The listing builds one solid part. Answer for the finished solid, in the listing's coordinates (mm). A direction names the side the tool comes from. Give positions to 0.01 mm unless a question says otherwise; leave off trailing zeros. Order: outer loops, then holes, each group sorted by start corner. A loop starts at its lowest first (then second) coordinate and runs counter-clockwise, first axis right, second up. Notation, with made-up numbers: (83, 53.5) - (115, 53.5) arc R6 cw to (115, 57.5) - close; hole circle Ø5 at (17, -8). An arc over 180 degrees is marked (long way). Write each question's results on one line, items separated by ' | '. Start each with the question number.
1. Section C-C (y = -38) is taken. Give the vertices of the cut face in (x, z).
2. Flat-ended cylindrical pins translate along their axes: pin 1 (4 mm diameter, centred on y = -10, z = 2.5, fed in from -X); pin 2 (5 mm diameter, centred on x = 0, y = -72.05, fed in from +Z); pin 3 (5 mm diameter, centred on x = 13, y = -22, fed in from +Z); pin 4 (6 mm diameter, centred on y = -20, z = -1, fed in from +X). Find the tip coordinate at first contact, or state that the pin passes through.
3. Section A-A (y = -15) is taken. Give the vertices of the cut face in (x, z).
4. Section B-B (x = -3) is taken. Give the vertices of the cut face in (y, z).
5. Find the intervals of material crossed by L1, parallel to Y at x = 0, z = 0.75; L2, parallel to Y at x = -15.5, z = 5; L3, parallel to Y at x = -8.5, z = -0.25, in increasing order.
6. Determine the mould class of faces 1 (the face through (-0.52, -68.08, -0.04)), 2 (the face through (2.305, -41.097, 0.035)), 3 (the face through (-19.33, -0.65, 0.04)), 4 (the face through (4, -33, -2.5)) for opening direction X: released by +X, released by -X, zero draft, split by the parting line, or undercut.
7. Which of the six approach directions +Z, -Z, +X, -X, +Y, -Y give full straight-line access (tool end or side, diameter ignored) to faces 5 (the face through (0.979, -37.367, 0.035)), 6 (the face through (-14, -9, 10)), 7 (the face through (-17.48, -8.8, 7.16))?
8. Section D-D (z = 3.5) is taken. State how many separate pieces and enclosed holes the cut face has, and give its area (3 significant figures).
from build123d import *

# Parameters (mm, degrees)
CROQUIS1_R              = 4
CROQUIS1_R_2            = 1.75
SALIENTE_EXTRUIR1_DEPTH = 2.5
CROQUIS1_3_R            = 2.5
CROQUIS1_3_R_2          = 1.75
SALIENTE_EXTRUIR2_DEPTH = 10
REDONDEO1_R             = 2
REDONDEO2_R             = 2


with BuildPart() as part:
    # Croquis1 → Saliente-Extruir1 (new, symmetric)
    with BuildSketch(Plane.XY):
        with BuildLine():
            Line((20.001432119, 0), (-20.001432119, 0))
            Line((-20.001432119, 0), (-14.963460754, -72.046347106))
            ThreePointArc((-14.963460754, -72.046347106), (0, -86), (14.963460754, -72.046347106))
            Line((14.963460754, -72.046347106), (20.001432119, 0))
        make_face()
        with Locations((0, -72.046347106)):
            Circle(CROQUIS1_R, mode=Mode.SUBTRACT)
        Polygon((12.515549555, -64.046347106), (-10.788577252, -64.046347106), (15.770666891, -17.496000466), align=None, mode=Mode.SUBTRACT)
        Polygon((-12.704099543, -61.349956664), (-16.011890152, -14.046347106), (14.28491785, -14.046347106), align=None, mode=Mode.SUBTRACT)
        with Locations((-15.5, -7.276347106)):
            Circle(CROQUIS1_R_2, mode=Mode.SUBTRACT)
        with Locations((15.5, -7.276347106)):
            Circle(CROQUIS1_R_2, mode=Mode.SUBTRACT)
    extrude(amount=SALIENTE_EXTRUIR1_DEPTH, both=True)

    # Croquis1_3 → Saliente-Extruir2 (add)
    # profile 1 of 2: a face of its own
    with BuildSketch(Plane.XY):
        with Locations((-15.5, -7.276347106)):
            Circle(CROQUIS1_3_R)
        with Locations((-15.5, -7.276347106)):
            Circle(CROQUIS1_3_R_2, mode=Mode.SUBTRACT)
    # profile 2 of 2: a face of its own
    with BuildSketch(Plane.XY):
        with Locations(Location((15.5, -7.276347106, 0), (0, 0, 180))):
            Circle(CROQUIS1_3_R)
        with Locations(Location((15.5, -7.276347106, 0), (0, 0, 180))):
            Circle(CROQUIS1_3_R_2, mode=Mode.SUBTRACT)
    extrude(amount=SALIENTE_EXTRUIR2_DEPTH)

    # Redondeo1
    redondeo1_edges = [part.edges().sort_by_distance(p)[0] for p in [
        (18, -7.276347106, 2.5),
        (-18, -7.276347106, 2.5),
    ]]
    fillet(redondeo1_edges, radius=REDONDEO1_R)

    # Redondeo2
    redondeo2_edges = [part.edges().sort_by_distance(p)[0] for p in [
        (-20.001432119, 0, 0),
        (20.001432119, 0, 0),
    ]]
    fillet(redondeo2_edges, radius=REDONDEO2_R)


solid = part.part
Reported:
1) outline: (-17.34, -2.5) - (-14.34, -2.5) - (-14.34, 2.5) - (-17.34, 2.5) - close; (0.62, -2.5) - (4.07, -2.5) - (4.07, 2.5) - (0.62, 2.5) - close; (14.34, -2.5) - (17.34, -2.5) - (17.34, 2.5) - (14.34, 2.5) - close
2) pin 1: x = -19.44 | pin 2: through | pin 3: z = 2.5 | pin 4: x = 18.81
3) outline: (-18.95, -2.5) - (-15.95, -2.5) - (-15.95, 2.5) - (-18.95, 2.5) - close; (13.74, -2.5) - (18.95, -2.5) - (18.95, 2.5) - (13.74, 2.5) - close
4) outline: (-85.7, -2.5) - (-74.69, -2.5) - (-74.69, 2.5) - (-85.7, 2.5) - close; (-69.4, -2.5) - (-64.05, -2.5) - (-64.05, 2.5) - (-69.4, 2.5) - close; (-50.4, -2.5) - (-44.34, -2.5) - (-44.34, 2.5) - (-50.4, 2.5) - close; (-14.05, -2.5) - (0, -2.5) - (0, 2.5) - (-14.05, 2.5) - close
5) L1: -86 to -76.05, -68.05 to -64.05, -45.14 to -39.08, -14.05 to 0 | L2: -9.78 to -9.03, -5.53 to -4.78 | L3: -83.36 to -64.05, -60.04 to -53.98, -14.05 to 0
6) face 1: undercut | face 2: undercut | face 3: released by -X | face 4: zero draft
7) face 5: +Z, -Z | face 6: +Z, +X, -X, +Y, -Y | face 7: +Z
8) separate pieces: 2 | enclosed holes: 2 | area: 28.8 mm²
